Design review of the part built by this model. Coordinates are the model's own, in mm. A direction names the side the tool comes from. Coordinates: 2 decimals unless noted, no trailing zeros. Write each loop counter-clockwise with the first axis right and the second up, starting at its lowest first coordinate (ties: lowest second). Pieces come first, ordered by that corner, then holes. Notation, with made-up numbers: (1.25, 80) -> (48.25, 80) arc R21 ccw to (48.25, 84) -> close; hole circle Ø1 at (-21, 10). An arc over 180 degrees is marked (long way). Answer in a Markdown table with one row per item. Add a question column.
Item 1: For faces 1 (the face through (-8.201, 62.464, 9.972)), 2 (the face through (30, -55, 3.3)), 3 (the face through (-17, 61, 12)), list the 3-axis set-ups (+Z, -Z, +X, -X, +Y, -Y) from which the entire face can be reached by the end or side of a thin tool; tool diameter is ignored.
Item 2: Take a section at A-A, the plane y = 0. Write out the cut boundary in (x, z).
Item 3: Clearance check with flat-ended pins moving along their axes: P1, Ø12, axis at x = 52.5, y = 27, coming from the -Z side; P2, Ø1, axis at y = -18.5, z = 1, coming from the +X side; P3, Ø1.5, axis at x = 50.5, y = 35, coming from the +Z side. State where each tip first meets the part, or that it passes through.
Item 4: Draft analysis for pull direction X (two halves, no side actions). For faces 4 (the face through (-9.764, 74.362, 5.916)), 5 (the face through (-67, 11, 0)), 6 (the face through (-59.94, 2.64, 6.48)), 7 (the face through (-8.071, 61.472, 4.138)), state which applies: released by +X, released by -X, zero draft, split by the parting line, or undercut.
Item 5: To check wall thickness, follow line 1 (Y direction, x = 0, z = 3.75); line 2 (Y direction, x = 0, z = 5.85); line 3 (X direction, y = 49.5, z = 8.25). State the ranges of each line that lie inside material, in increasing order.
from build123d import *

# Parameters (mm, degrees)
SKETCH_1_R           = 75
SKETCH_1_R_2         = 67.5
F_01_CASE_D135_DEPTH = 3.3
SKETCH_2_R           = 75
SKETCH_2_R_2         = 62
F_02_LIP_CONE_DEPTH  = 1.7
SKETCH_3_R           = 75
SKETCH_3_R_2         = 60
F_03_LIP_D120_DEPTH  = 3
SKETCH_4_R           = 75
SKETCH_4_R_2         = 63
F_04_DUST_LIP_DEPTH  = 4


with BuildPart() as part:
    # 草图1 → 01_CASE_D135 (new body)
    with BuildSketch(Plane.XY):
        Circle(SKETCH_1_R)
        Circle(SKETCH_1_R_2, mode=Mode.SUBTRACT)
    extrude(amount=F_01_CASE_D135_DEPTH)

    # 草图2 → 02_LIP_CONE (add)
    with BuildSketch(Plane.XY.offset(3.3)):
        Circle(SKETCH_2_R)
        Circle(SKETCH_2_R_2, mode=Mode.SUBTRACT)
    extrude(amount=F_02_LIP_CONE_DEPTH)

    # 草图3 → 03_LIP_D120 (add)
    with BuildSketch(Plane.XY.offset(5)):
        Circle(SKETCH_3_R)
        Circle(SKETCH_3_R_2, mode=Mode.SUBTRACT)
    extrude(amount=F_03_LIP_D120_DEPTH)

    # 草图4 → 04_DUST_LIP (add)
    with BuildSketch(Plane.XY.offset(8)):
        Circle(SKETCH_4_R)
        Circle(SKETCH_4_R_2, mode=Mode.SUBTRACT)
    extrude(amount=F_04_DUST_LIP_DEPTH)


solid = part.part
Answers:
| question | item | result |
|---|---|---|
| 1 | face 1 | +Z |
| 1 | face 2 | -Z |
| 1 | face 3 | +Z, +X, -X, +Y, -Y |
| 2 | outline | (-75, 0) -> (-67.5, 0) -> (-67.5, 3.3) -> (-62, 3.3) -> (-62, 5) -> (-60, 5) -> (-60, 8) -> (-63, 8) -> (-63, 12) -> (-75, 12) -> close; (60, 5) -> (62, 5) -> (62, 3.3) -> (67.5, 3.3) -> (67.5, 0) -> (75, 0) -> (75, 12) -> (63, 12) -> (63, 8) -> (60, 8) -> close |
| 3 | P1 | stops at z = 3.3 |
| 3 | P2 | stops at x = 72.81 |
| 3 | P3 | stops at z = 8 |
| 4 | face 4 | split by the parting line |
| 4 | face 5 | zero draft |
| 4 | face 6 | undercut |
| 4 | face 7 | undercut |
| 5 | line 1 | y = -75 to -62, 62 to 75 |
| 5 | line 2 | y = -75 to -60, 60 to 75 |
| 5 | line 3 | x = -56.34 to -38.97, 38.97 to 56.34 |
